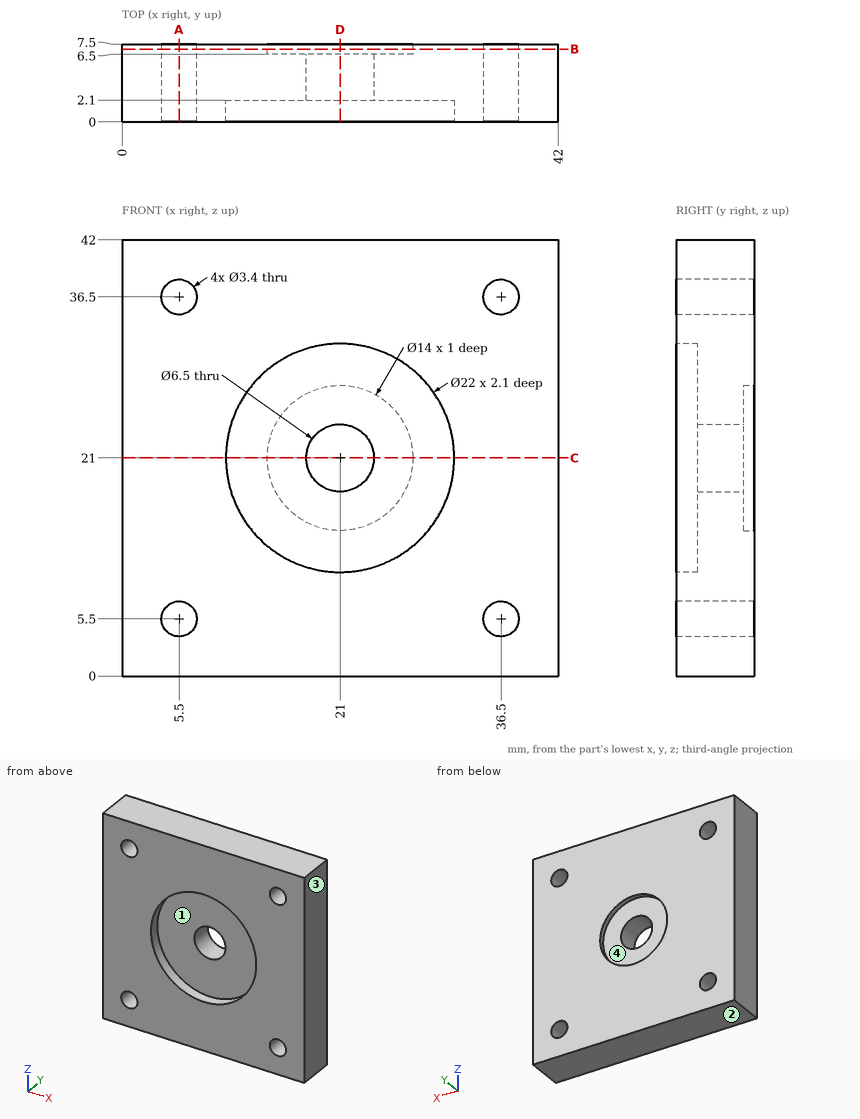
Geometry: see drawing. Coordinates: mm, zero at the bounding-box minimum. Round coordinates to 2 decimals unless told otherwise and drop trailing zeros. Write each loop counter-clockwise with the first axis right and the second up, starting at its lowest first coordinate (ties: lowest second). Pieces come first, ordered by that corner, then holes.
Item 1: Section query D-D (x = 21). Return loops of the section in (y, z).
Item 2: Pin query (flat end, axial travel): P1, Ø11, axis at x = 21, z = 21, coming from the +Y side; P2, Ø17.5, axis at x = 21, z = 21, coming from the -Y side. Return the tip coordinate at first contact, or that it passes through.
Item 3: Section query B-B (y = 7). Return loops of the section in (x, z).
Item 4: Section query A-A (x = 5.5). Return loops of the section in (y, z).
Item 5: Material intervals for L1, parallel to Z at x = 5.5, y = 5.75; L2, parallel to X at y = 3.25, z = 35, sorted ascending.
Item 6: Mould query, pull axis X, two halves, no side actions, for the marked faces 1, 2, 3 and 4. Classes: +X half, -X half, draft (parallel to the pull), parting line (faces both ways), or undercut.
Item 7: Section query C-C (z = 21). Return loops of the section in (x, y), plus the area to 3 significant figures.
Completed:
1. outline: (0, 0) - (7.5, 0) - (7.5, 14) - (6.5, 14) - (6.5, 17.75) - (2.1, 17.75) - (2.1, 10) - (0, 10) - close; (0, 32) - (2.1, 32) - (2.1, 24.25) - (6.5, 24.25) - (6.5, 28) - (7.5, 28) - (7.5, 42) - (0, 42) - close
2. P1: stops at y = 6.5
2. P2: stops at y = 2.1
3. outline: (0, 0) - (42, 0) - (42, 42) - (0, 42) - close; hole circle Ø3.4 at (5.5, 5.5); hole circle Ø3.4 at (5.5, 36.5); hole circle Ø14 at (21, 21); hole circle Ø3.4 at (36.5, 5.5); hole circle Ø3.4 at (36.5, 36.5)
4. outline: (0, 0) - (7.5, 0) - (7.5, 3.8) - (0, 3.8) - close; (0, 7.2) - (7.5, 7.2) - (7.5, 34.8) - (0, 34.8) - close; (0, 38.2) - (7.5, 38.2) - (7.5, 42) - (0, 42) - close
5. L1: z = 0 to 3.8, 7.2 to 34.8, 38.2 to 42
5. L2: x = 0 to 4.7, 6.3 to 35.7, 37.3 to 42
6. face 1: undercut
6. face 2: draft
6. face 3: +X half
6. face 4: undercut
7. outline: (0, 0) - (10, 0) - (10, 2.1) - (17.75, 2.1) - (17.75, 6.5) - (14, 6.5) - (14, 7.5) - (0, 7.5) - close; (24.25, 2.1) - (32, 2.1) - (32, 0) - (42, 0) - (42, 7.5) - (28, 7.5) - (28, 6.5) - (24.25, 6.5) - close
7. area: 226 mm2
